For this review, use the dimensioned drawing (mm, ordinates from the lowest corner) and the shaded views. A direction names the side the tool comes from. Coordinates: 2 decimals unless noted, no trailing zeros. Loops run counter-clockwise (first coordinate to the right, second up) from the corner with the lowest first, then second, coordinate; pieces in that order, holes last. Notation, with made-up numbers: M 66,36.25 L 114,36.25 A21 cw 114,66.25 Z; hole C 63,-36.75 d5. An arc over 180 degrees is marked long. Write item = value, one per line. Start each with the question number.
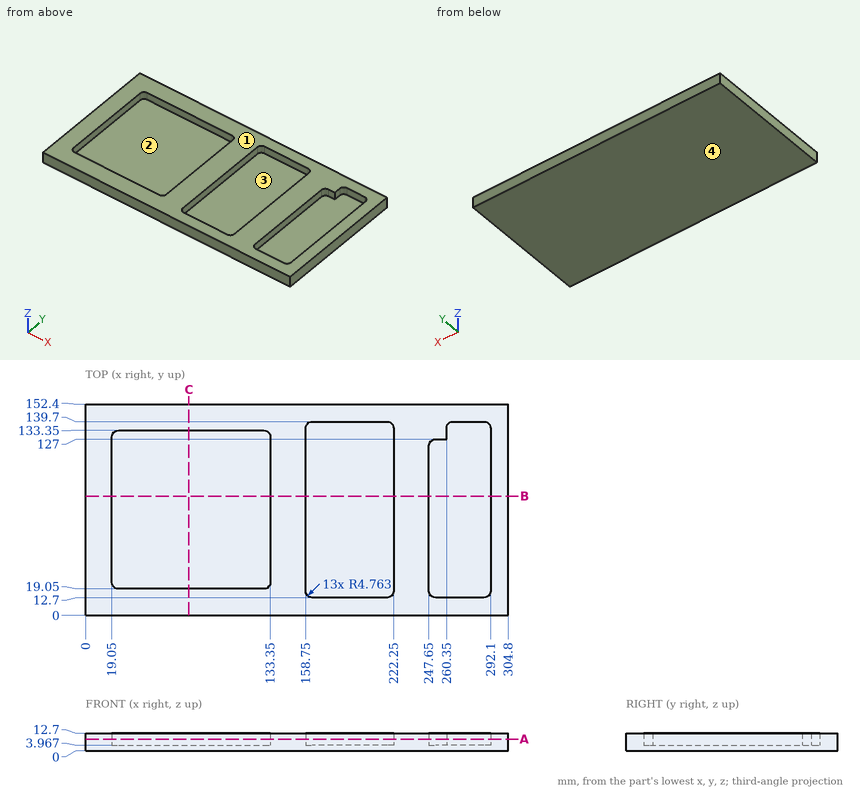
Q1. Mouldability with a two-part tool opening along X and no side actions: class the marked faces 1 and 2 as released by +X, released by -X, zero draft, split by the parting line, or undercut.
Q2. Clearance check with a flat-ended pin moving along its axis: P1, Ø19, axis at x = 196.5, y = 87.5, coming from the +Z side. State where the tip first meets the part, or that it passes through.
Q3. Add section A-A on z = 8.5. Give the number of separate pieces and of enclosed holes in the cut face, plus the area to 3 significant figures.
Q4. To check wall thickness, follow line 1 (X direction, y = 65, z = 4); line 2 (Y direction, x = 187.5, z = 4); line 3 (Y direction, x = 109, z = 8.25). State the ranges of each line that lie inside material, in increasing order. Write a range as from..to.
Q5. Add section B-B on y = 86. State the section outline as (x, z) points, plus the area to 3 significant figures.
Q6. For the marked faces 3 and 4, list the 3-axis set-ups (+Z, -Z, +X, -X, +Y, -Y) from which the entire face can be reached by the end or side of a thin tool; tool diameter is ignored.
Q7. Add section C-C on x = 74.5. State the section outline as (y, z) points.
Values follow:
q1.face_1 = zero draft
q1.face_2 = undercut
q2.P1 = 3.97
q3.separate_pieces = 1
q3.enclosed_holes = 3
q3.area = 19,900 mm2
q4.line_1 = 0..19.05, 133.35..158.75, 222.25..247.65, 292.1..304.8
q4.line_2 = 0..12.7, 139.7..152.4
q4.line_3 = 0..19.05, 133.35..152.4
q5.outline = M 0,0 L 304.8,0 L 304.8,12.7 L 292.1,12.7 L 292.1,3.97 L 247.65,3.97 L 247.65,12.7 L 222.25,12.7 L 222.25,3.97 L 158.75,3.97 L 158.75,12.7 L 133.35,12.7 L 133.35,3.97 L 19.05,3.97 L 19.05,12.7 L 0,12.7 Z
q5.area = 1,930 mm2
q6.face_3 = +Z
q6.face_4 = -Z, +X, -X, +Y, -Y
q7.outline = M 0,0 L 152.4,0 L 152.4,12.7 L 133.35,12.7 L 133.35,3.97 L 19.05,3.97 L 19.05,12.7 L 0,12.7 Z
